Could you check a few things on this drawing? It's one solid part, dimensions in mm from its lowest x, y, z. A direction names the side the tool comes from. Round coordinates to 2 decimals unless told otherwise and drop trailing zeros. Loops run counter-clockwise (first coordinate to the right, second up) from the corner with the lowest first, then second, coordinate; pieces in that order, holes last. Notation, with made-up numbers: M 87,35 L 116,35 A20 cw 116,64 Z; hole C -3.5,3 d9. An arc over 180 degrees is marked long. Return JSON: item names as keys, results as strings.
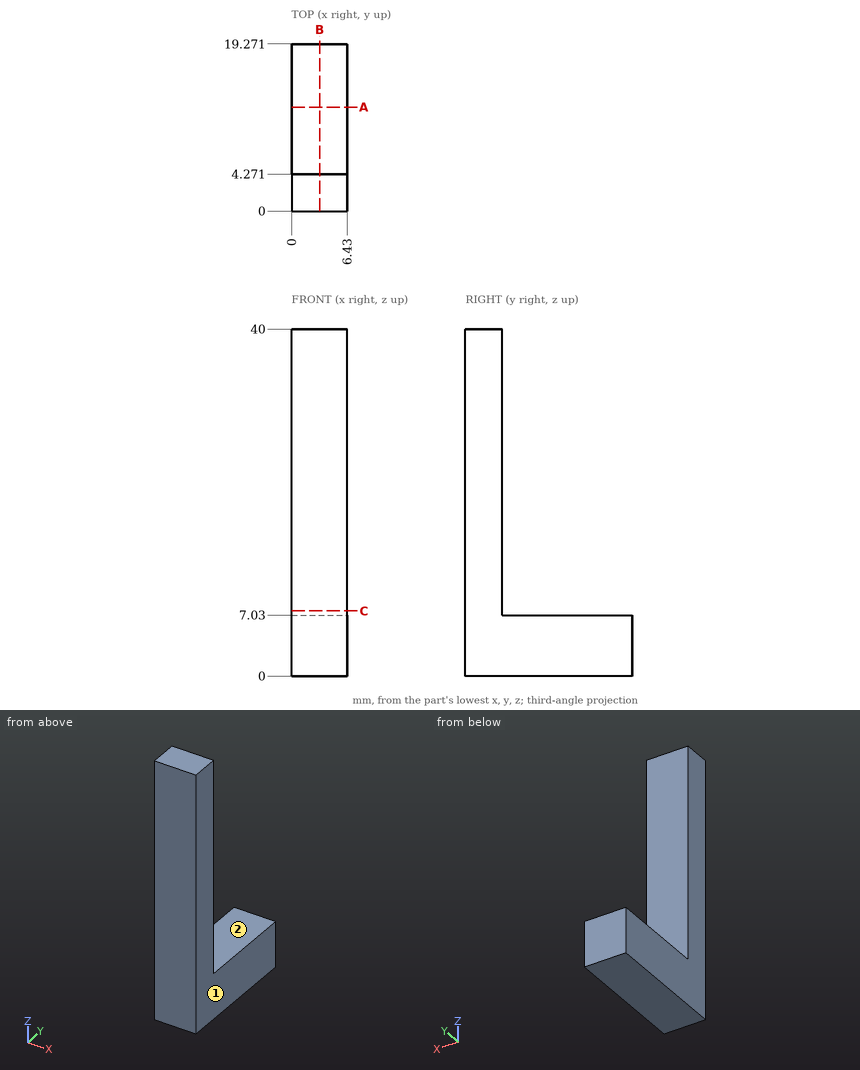
Q1. Suppose I cut it at A-A, the plane y = 12. Please give me the cut outline in (x, z).
Results:
{"outline": "M 0,0 L 6.43,0 L 6.43,7.03 L 0,7.03 Z"}
Q2. Suppose I cut it at C-C, the plane z = 7.5. Please give me the cut outline in (x, y).
Results:
{"outline": "M 0,0 L 6.43,0 L 6.43,4.27 L 0,4.27 Z"}
Q3. Suppose I cut it at B-B, the plane x = 3.25. Please give me the cut outline in (y, z).
Results:
{"outline": "M 0,0 L 19.27,0 L 19.27,7.03 L 4.27,7.03 L 4.27,40 L 0,40 Z"}
Q4. On a 3-axis mill with a long thin cutter (end or side, diameter ignored), from which of +Z, -Z, +X, -X, +Y, -Y can I reach the whole of each face in a straight line? I mean the marked faces 1 and 2. Say none if no direction works.
Results:
{"face 1": "+Z, -Z, +X, +Y, -Y", "face 2": "+Z, +X, -X, +Y"}
Q5. If I drill on line 1 along Y through (x, z) = (3.5, 19); line 2 along Z through (x, y) = (4.5, 13.5), over which ranges is the centre line in solid material (lowest first)?
Results:
{"line 1": "y = 0 to 4.27", "line 2": "z = 0 to 7.03"}
Q6. I'm going to push a flat-ended pin straight in: pin 1 Ø1.5 at (x, y) = (5, 9) entering from +Z. Where does the tip first touch, or does it pass through?
Results:
{"pin 1": "stops at z = 7.03"}
